Verification items for the finished model (mm, model axes). Give positions to 0.01 mm unless a question says otherwise; leave off trailing zeros.
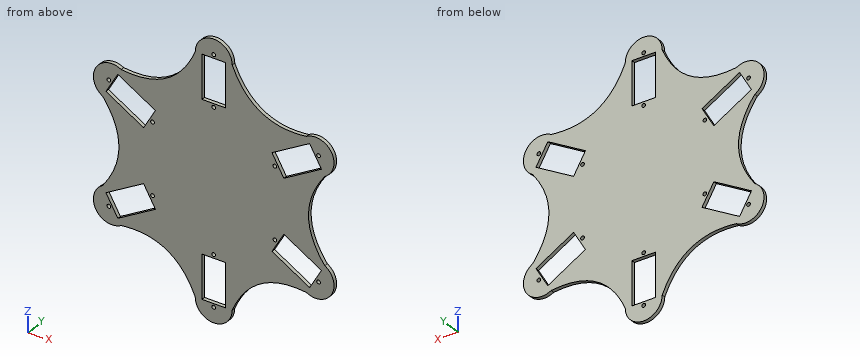
from build123d import *

# Parameters (mm, degrees)
SKETCH4_W           = 12.8
SKETCH4_H           = 23.5
SKETCH4_R           = 1
BOSS_EXTRUDE3_DEPTH = 2


with BuildPart() as part:
    # Sketch4 → Boss-Extrude3 (new body)
    with BuildSketch(Plane(origin=(0, 0, 0), x_dir=(1, 0, 0), z_dir=(0, 1, 0))):
        with BuildLine():
            ThreePointArc((10, 63.612159322), (0, 73.612159322), (-10, 63.612159322))
            add(Edge.make_bspline(
                [(-10, 63.612159322), (-21.25, 36.806079661), (-50.089745962, 40.466333699)],
                knots=[0, 0, 0, 1, 1, 1], degree=2))
            ThreePointArc((-50.089745962, 40.466333699), (-63.75, 36.806079661), (-60.089745962, 23.145825623))
            add(Edge.make_bspline(
                [(-60.089745962, 23.145825623), (-42.5, 0), (-60.089745962, -23.145825623)],
                knots=[0, 0, 0, 1, 1, 1], degree=2))
            ThreePointArc((-60.089745962, -23.145825623), (-63.75, -36.806079661), (-50.089745962, -40.466333699))
            add(Edge.make_bspline(
                [(-50.089745962, -40.466333699), (-21.25, -36.806079661), (-10, -63.612159322)],
                knots=[0, 0, 0, 1, 1, 1], degree=2))
            ThreePointArc((-10, -63.612159322), (0, -73.612159322), (10, -63.612159322))
            add(Edge.make_bspline(
                [(10, -63.612159322), (21.25, -36.806079661), (50.089745962, -40.466333699)],
                knots=[0, 0, 0, 1, 1, 1], degree=2))
            ThreePointArc((50.089745962, -40.466333699), (63.75, -36.806079661), (60.089745962, -23.145825623))
            add(Edge.make_bspline(
                [(60.089745962, -23.145825623), (42.5, 0), (60.089745962, 23.145825623)],
                knots=[0, 0, 0, 1, 1, 1], degree=2))
            ThreePointArc((60.089745962, 23.145825623), (63.75, 36.806079661), (50.089745962, 40.466333699))
            add(Edge.make_bspline(
                [(50.089745962, 40.466333699), (21.25, 36.806079661), (10, 63.612159322)],
                knots=[0, 0, 0, 1, 1, 1], degree=2))
        make_face()
        with Locations((0, -51.862159322)):
            Rectangle(SKETCH4_W, SKETCH4_H, mode=Mode.SUBTRACT)
        Polygon((31.538148973, -25.598642245), (37.938148973, -14.513517077), (58.289745962, -26.263517077), (51.889745962, -37.348642245), align=None, mode=Mode.SUBTRACT)
        Polygon((-37.938148973, -14.513517077), (-31.538148973, -25.598642245), (-51.889745962, -37.348642245), (-58.289745962, -26.263517077), align=None, mode=Mode.SUBTRACT)
        with Locations((0, 51.862159322)):
            Rectangle(SKETCH4_W, SKETCH4_H, mode=Mode.SUBTRACT)
        with Locations((0, 65.512159322)):
            Circle(SKETCH4_R, mode=Mode.SUBTRACT)
        Polygon((31.538148973, 25.598642245), (51.889745962, 37.348642245), (58.289745962, 26.263517077), (37.938148973, 14.513517077), align=None, mode=Mode.SUBTRACT)
        Polygon((-37.938148973, 14.513517077), (-58.289745962, 26.263517077), (-51.889745962, 37.348642245), (-31.538148973, 25.598642245), align=None, mode=Mode.SUBTRACT)
        with Locations((33.092700706, 19.106079661)):
            Circle(SKETCH4_R, mode=Mode.SUBTRACT)
        with Locations((0, 38.212159322)):
            Circle(SKETCH4_R, mode=Mode.SUBTRACT)
        with Locations((-33.092700706, -19.106079661)):
            Circle(SKETCH4_R, mode=Mode.SUBTRACT)
        with Locations((0, -38.212159322)):
            Circle(SKETCH4_R, mode=Mode.SUBTRACT)
        with Locations((33.092700706, -19.106079661)):
            Circle(SKETCH4_R, mode=Mode.SUBTRACT)
        with Locations((-33.092700706, 19.106079661)):
            Circle(SKETCH4_R, mode=Mode.SUBTRACT)
        with Locations((56.735194229, 32.756079661)):
            Circle(SKETCH4_R, mode=Mode.SUBTRACT)
        with Locations((-56.735194229, 32.756079661)):
            Circle(SKETCH4_R, mode=Mode.SUBTRACT)
        with Locations((-56.735194229, -32.756079661)):
            Circle(SKETCH4_R, mode=Mode.SUBTRACT)
        with Locations((56.735194229, -32.756079661)):
            Circle(SKETCH4_R, mode=Mode.SUBTRACT)
        with Locations((0, -65.512159322)):
            Circle(SKETCH4_R, mode=Mode.SUBTRACT)
    extrude(amount=BOSS_EXTRUDE3_DEPTH)


solid = part.part
(1) Section check A-A, the plane y = 0.55. Give the number of separate pieces and of enclosed holes in the cut face, then the cut area to 3 significant figures.
Solved:
separate pieces: 1
enclosed holes: 18
area: 9,630 mm2
(2) Go/stop test with flat-tipped pins: pin 1 (1 mm diameter, centred on y = 1, z = -55, fed in from +X); pin 2 (0.6 mm diameter, centred on x = 2.5, y = 1, fed in from -Z); pin 3 (1 mm diameter, centred on y = 1, z = 53, fed in from +X). Record where each tip stops, or that it passes through.
Solved:
pin 1: stops at x = 14.93
pin 2: stops at z = -73.37
pin 3: stops at x = 16.41
(3) Scan lines: line 1 (X direction, y = 1, z = -50.5); line 2 (X direction, y = 1.7, z = -36); line 3 (Z direction, x = 43, y = 1.15). Record each from-to range of solid material in increasing order.
Solved:
line 1: x = -18.12 to -6.4, 6.4 to 18.12
line 2: x = -64.17 to -52.67, -49.55 to 49.55, 52.67 to 64.17
line 3: z = -40.03 to -32.22, -17.44 to 17.44, 32.22 to 40.03
